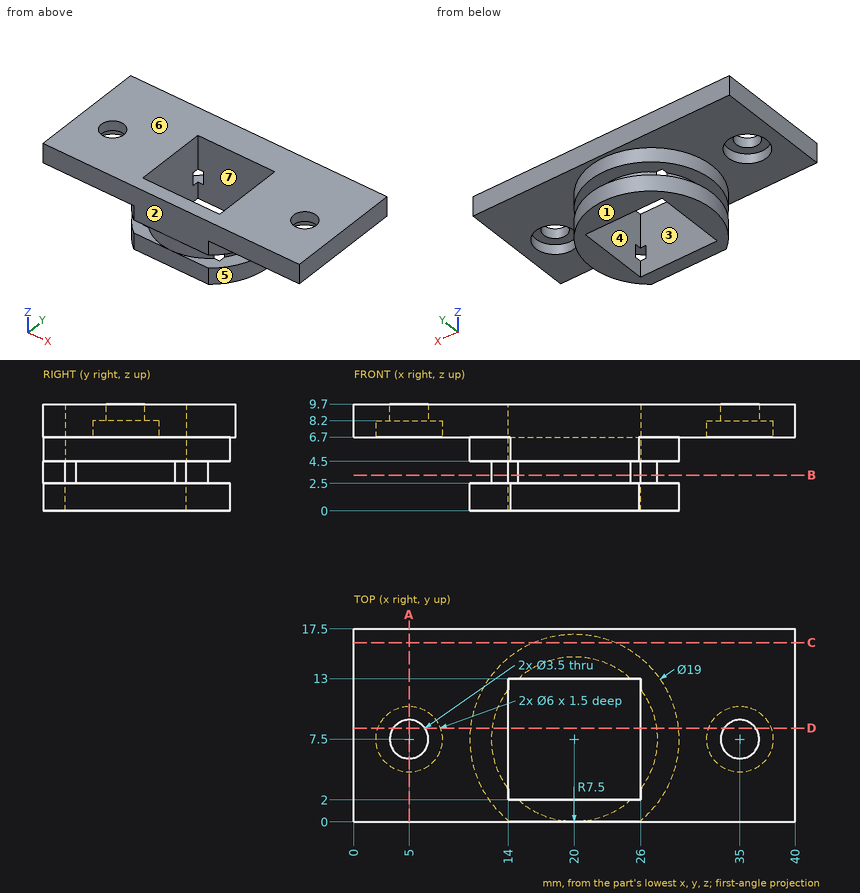
Print and shaded views of the part. All mm, measured from the part's lowest x, y and z. A direction names the side the tool comes from. Give positions to 0.01 mm unless a question says otherwise; leave off trailing zeros. Loops run counter-clockwise (first coordinate to the right, second up) from the corner with the lowest first, then second, coordinate; pieces in that order, holes last. Notation, with made-up numbers: (-26, 1) -> (-10, 1) arc R25 ccw to (-10, 38) -> close; hole circle Ø10 at (2.25, 7.5). An arc over 180 degrees is marked (long way). Use CSV: the item, a comma, the result in double quotes. Start each with the question number.
1) Tool access for the marked faces 5, 6 and 7: list every direction of +Z, -Z, +X, -X, +Y, -Y with a clear straight run to the whole face (end or side of a thin tool).
2) Slice it at B-B on z = 3.25. Give the cut face in (x, y).
3) Slice it at D-D on y = 8.5. Give the number of separate pieces and of enclosed holes in the cut face, plus the area to 3 significant figures.
4) Wall check: line 1 (Y direction, x = 35, z = 7.3); line 2 (Y direction, x = 5, z = 9.4); line 3 (Z direction, x = 31, y = 5). Give the ranges that are in metal, low to high.
5) Flat gauge pins, fed straight in: pin 1 Ø3 at (x, z) = (22, 4) entering from -Y; pin 2 Ø6.5 at (x, y) = (6, 8.5) entering from -Z; pin 3 Ø1.5 at (x, z) = (24, 5) entering from +Y; pin 4 Ø5 at (x, y) = (35, 7.5) entering from -Z. Where does each tip first touch, or does it go through?
6) Slice it at A-A on x = 5. Give the cut face in (y, z), plus the area to 4 significant figures.
7) Mould opens along Y. For the marked faces 1, 2, 3 and 4 say: released by +Y, released by -Y, zero draft, split by the parting line, or undercut.
8) Slice it at C-C on y = 16.25. Give the cut face in (x, z), plus the area to 3 significant figures.
Computed values:
1,face 5,"-Z"
1,face 6,"+Z, +X, -X, +Y, -Y"
1,face 7,"+Z, -Z"
2,outline,"(14, 3) -> (14, 12) arc R7.5 ccw to start; (14.9, 2) arc R7.5 ccw to (25.1, 2) -> close; (14.9, 13) -> (25.1, 13) arc R7.5 ccw to start; (26, 3) arc R7.5 ccw to (26, 12) -> close"
3,separate pieces,"4"
3,enclosed holes,"0"
3,area,"96.5 mm^2"
4,line 1,"y = 0 to 4.5, 10.5 to 17.5"
4,line 2,"y = 0 to 5.75, 9.25 to 17.5"
4,line 3,"z = 6.7 to 9.7"
5,pin 1,"stops at y = 0"
5,pin 2,"stops at z = 6.7"
5,pin 3,"stops at y = 16.43"
5,pin 4,"stops at z = 8.2"
6,outline,"(0, 6.7) -> (4.5, 6.7) -> (4.5, 8.2) -> (5.75, 8.2) -> (5.75, 9.7) -> (0, 9.7) -> close; (9.25, 8.2) -> (10.5, 8.2) -> (10.5, 6.7) -> (17.5, 6.7) -> (17.5, 9.7) -> (9.25, 9.7) -> close"
6,area,"38.25 mm^2"
7,face 1,"zero draft"
7,face 2,"released by -Y"
7,face 3,"undercut"
7,face 4,"undercut"
8,outline,"(0, 6.7) -> (16.3, 6.7) -> (16.3, 4.5) -> (23.7, 4.5) -> (23.7, 6.7) -> (40, 6.7) -> (40, 9.7) -> (0, 9.7) -> close; (16.3, 0) -> (23.7, 0) -> (23.7, 2.5) -> (16.3, 2.5) -> close"
8,area,"155 mm^2"
